```python
from build123d import *

# Parameters (mm, degrees)
SZKIC1_W                         = 42
SZKIC1_H                         = 42
DODANIE_WYCI_GNI_CIE1_DEPTH      = 39
SZKIC1_3_R                       = 18
DODANIE_WYCI_GNI_CIE2_DEPTH      = 62.5
SZKIC1_4_R                       = 11
DODANIE_WYCI_GNI_CIE3_DEPTH      = 64.5
SZKIC1_5_R                       = 4
DODANIE_WYCI_GNI_CIE4_DEPTH      = 66.8
DODANIE_WYCI_GNI_CIE5_DEPTH      = 82
SZKIC2_OUTSIDE_W                 = 64.25
SZKIC2_OUTSIDE_H                 = 64.25
SZKIC2_OUTSIDE_R                 = 26.85
WYTNIJ_WYCI_GNI_CIE2_DEPTH       = 83
WYTNIJ_WYCI_GNI_CIE3_START       = 8.9
SZKIC3_OUTSIDE_W                 = 64.25
SZKIC3_OUTSIDE_H                 = 64.25
SZKIC3_OUTSIDE_R                 = 25.1
WYTNIJ_WYCI_GNI_CIE3_DEPTH       = 17
SZKIC4_R                         = 4.65
WYTNIJ_WYCI_GNI_CIE5_DEPTH       = 4
OTW_R_GWINTOWANY_M31_D           = 2.5
OTW_R_GWINTOWANY_M31_DEPTH       = 9
OTW_R_GWINTOWANY_M31_CSINK_D     = 3
OTW_R_GWINTOWANY_M31_CSINK_ANGLE = 90
OTW_R_GWINTOWANY_M31_TIP         = 0.751075774
DODANIE_WYCI_GNI_CIE6_START      = 21
SZKIC18_W                        = 16.4
SZKIC18_H                        = 9.4
DODANIE_WYCI_GNI_CIE6_DEPTH      = 6


with BuildPart() as part:
    # Szkic1 → Dodanie-wyci_gni_cie1 (new body)
    with BuildSketch(Plane(origin=(0, 0, 0), x_dir=(1, 0, 0), z_dir=(0, 1, 0))):
        Rectangle(SZKIC1_W, SZKIC1_H)
    extrude(amount=DODANIE_WYCI_GNI_CIE1_DEPTH)

    # Szkic1_3 → Dodanie-wyci_gni_cie2 (add)
    with BuildSketch(Plane(origin=(0, 0, 0), x_dir=(1, 0, 0), z_dir=(0, 1, 0))):
        Circle(SZKIC1_3_R)
    extrude(amount=DODANIE_WYCI_GNI_CIE2_DEPTH)

    # Szkic1_4 → Dodanie-wyci_gni_cie3 (add)
    with BuildSketch(Plane(origin=(0, 0, 0), x_dir=(1, 0, 0), z_dir=(0, 1, 0))):
        Circle(SZKIC1_4_R)
    extrude(amount=DODANIE_WYCI_GNI_CIE3_DEPTH)

    # Szkic1_5 → Dodanie-wyci_gni_cie4 (add)
    with BuildSketch(Plane(origin=(0, 0, 0), x_dir=(1, 0, 0), z_dir=(0, 1, 0))):
        Circle(SZKIC1_5_R)
    extrude(amount=DODANIE_WYCI_GNI_CIE4_DEPTH)

    # Szkic1_6 → Dodanie-wyci_gni_cie5 (add)
    with BuildSketch(Plane(origin=(0, 0, 0), x_dir=(1, 0, 0), z_dir=(0, 1, 0))):
        with BuildLine():
            Line((-2.645751311, -3), (2.645751311, -3))
            ThreePointArc((2.645751311, -3), (0, 4), (-2.645751311, -3))
        make_face()
    extrude(amount=DODANIE_WYCI_GNI_CIE5_DEPTH)

    # Szkic2 outside → Wytnij-wyci_gni_cie2 (cut, through all)
    with BuildSketch(Plane(origin=(0, 0, 0), x_dir=(1, 0, 0), z_dir=(0, 1, 0))):
        Rectangle(SZKIC2_OUTSIDE_W, SZKIC2_OUTSIDE_H)
        Circle(SZKIC2_OUTSIDE_R, mode=Mode.SUBTRACT)
    extrude(amount=WYTNIJ_WYCI_GNI_CIE2_DEPTH, mode=Mode.SUBTRACT)

    # Szkic3 outside → Wytnij-wyci_gni_cie3 (cut)
    with BuildSketch(Plane(origin=(0, 0, 0), x_dir=(1, 0, 0), z_dir=(0, 1, 0)).offset(WYTNIJ_WYCI_GNI_CIE3_START)):
        Rectangle(SZKIC3_OUTSIDE_W, SZKIC3_OUTSIDE_H)
        Circle(SZKIC3_OUTSIDE_R, mode=Mode.SUBTRACT)
    extrude(amount=WYTNIJ_WYCI_GNI_CIE3_DEPTH, mode=Mode.SUBTRACT)

    # Szkic4 → Wytnij-wyci_gni_cie5 (cut)
    with BuildSketch(Plane(origin=(0, 0, 0), x_dir=(1, 0, 0), z_dir=(0, 1, 0))):
        Circle(SZKIC4_R)
    extrude(amount=WYTNIJ_WYCI_GNI_CIE5_DEPTH, mode=Mode.SUBTRACT)

    # Otw_r gwintowany M31
    with Locations(Plane(origin=(0, 62.5, 0), x_dir=(1, 0, 0), z_dir=(0, 1, 0))):
        with Locations((-10.606601718, 10.606601718), (10.606601718, 10.606601718), (10.606601718, -10.606601718), (-10.606601718, -10.606601718)):
            CounterSinkHole(OTW_R_GWINTOWANY_M31_D / 2, OTW_R_GWINTOWANY_M31_CSINK_D / 2, depth=OTW_R_GWINTOWANY_M31_DEPTH, counter_sink_angle=OTW_R_GWINTOWANY_M31_CSINK_ANGLE)
            with Locations((0, 0, -(OTW_R_GWINTOWANY_M31_DEPTH + OTW_R_GWINTOWANY_M31_TIP / 2))):  # 118° drill point
                Cone(0, OTW_R_GWINTOWANY_M31_D / 2, OTW_R_GWINTOWANY_M31_TIP, mode=Mode.SUBTRACT)

    # Szkic18 → Dodanie-wyci_gni_cie6 (add)
    with BuildSketch(Plane.XY.offset(DODANIE_WYCI_GNI_CIE6_START)):
        with Locations((0, 4.7)):
            Rectangle(SZKIC18_W, SZKIC18_H)
    extrude(amount=DODANIE_WYCI_GNI_CIE6_DEPTH)


solid = part.part
```
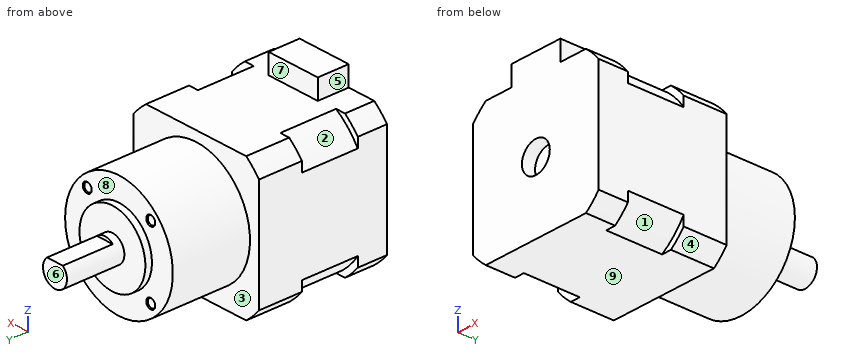
Geometry check sheet. Reference: the model listing, model coordinates, mm. Face numbers are marked on the shaded views. A direction names the side the tool comes from. Coordinates: 2 decimals unless noted, no trailing zeros. Write each loop counter-clockwise with the first axis right and the second up, starting at its lowest first coordinate (ties: lowest second). Pieces come first, ordered by that corner, then holes. Notation, with made-up numbers: M 60,88 L 95,88 A20 ccw 95,111 Z; hole C 43,-8 d5. An arc over 180 degrees is marked long. Use one line per item in the form item = value. Start each with the question number.
1) Go/stop test with flat-tipped pins: pin 1 Ø12 at (x, z) = (-8.5, -7.5) entering from +Y; pin 2 Ø6.5 at (y, z) = (2.5, 24) entering from -X; pin 3 Ø6 at (x, z) = (16.5, -18) entering from +Y. Record where each tip stops, or that it passes through.
2) Section check B-B on y = 21. Enter the section's corners in (x, z).
3) Thickness scan on probe 1 along X at (y, z) = (2, 0); probe 2 along Y at (x, z) = (-19, 18); probe 3 along Y at (x, z) = (-9, -10.5). Record the ranges inside material, lowest first. Write a range as from..to.
4) Release check for a two-part mould opening along Y. For the marked faces 1, 2, 3 and 4 record: pulls with the +Y half, pulls with the -Y half, needs draft (parallel to the pull), parting line crosses it, or undercut.
5) Section check D-D on y = 75. Enter the section's corners in (x, z).
6) Section check A-A on x = 0. Enter the section's corners in (y, z), and give its area (3 significant figures).
7) Set-up check for the marked faces 5, 6, 7, 8 and 9: record each of +Z, -Z, +X, -X, +Y, -Y from which the full face is reachable in a straight line by a thin tool's end or side.
8) Section check C-C on y = 55. Enter the section's corners in (x, z).
Responses:
q1.pin_1 = 64.5
q1.pin_2 = -17.04
q1.pin_3 = 39
q2.outline = M -21,-13.75 A25.1 ccw -13.75,-21 L 13.75,-21 A25.1 ccw 21,-13.75 L 21,13.75 A25.1 ccw 13.75,21 L -13.75,21 A25.1 ccw -21,13.75 Z
q3.probe_1 = -21..-4.65, 4.65..21
q3.probe_2 = 0..8.9, 25.9..39
q3.probe_3 = 0..62.5
q4.face_1 = undercut
q4.face_2 = undercut
q4.face_3 = pulls with the +Y half
q4.face_4 = needs draft
q5.outline = M -2.65,3 A4 ccw long 2.65,3 Z
q6.outline = M 0,-21 L 39,-21 L 39,-18 L 62.5,-18 L 62.5,-11 L 64.5,-11 L 64.5,-4 L 82,-4 L 82,3 L 66.8,3 L 66.8,4 L 64.5,4 L 64.5,11 L 62.5,11 L 62.5,18 L 39,18 L 39,21 L 9.4,21 L 9.4,27 L 0,27 L 0,4.65 L 4,4.65 L 4,-4.65 L 0,-4.65 Z
q6.area = 2,670 mm2
q7.face_5 = +Z, -X, +Y, -Y
q7.face_6 = +Z, -Z, +X, -X, +Y
q7.face_7 = +Z, +X, -X, +Y
q7.face_8 = +Y
q7.face_9 = -Z, +X, -X, +Y, -Y
q8.outline = C 0,0 d36; hole C -10.61,-10.61 d2.5; hole C -10.61,10.61 d2.5; hole C 10.61,-10.61 d2.5; hole C 10.61,10.61 d2.5
